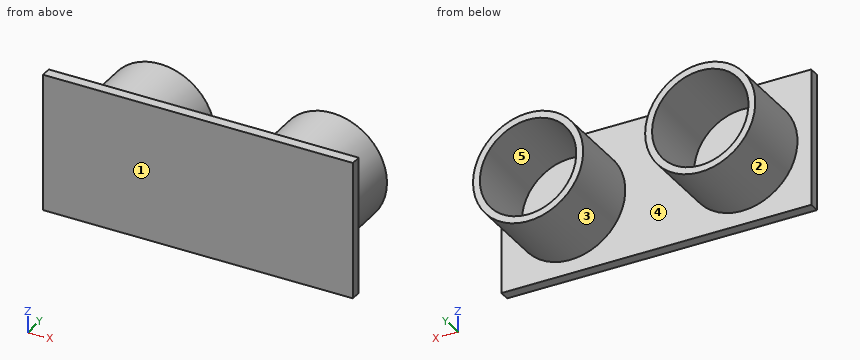
```python
from build123d import *

# Parameters (mm, degrees)
SKETCH1_W           = 45
SKETCH1_H           = 20
BOSS_EXTRUDE1_DEPTH = 1.5
SKETCH3_R           = 8
SKETCH3_R_2         = 7
BOSS_EXTRUDE2_DEPTH = 11


with BuildPart() as part:
    # Sketch1 → Boss-Extrude1 (new body)
    with BuildSketch(Plane(origin=(0, 0, 0), x_dir=(1, 0, 0), z_dir=(0, 1, 0))):
        Rectangle(SKETCH1_W, SKETCH1_H)
    extrude(amount=BOSS_EXTRUDE1_DEPTH)

    # Sketch3 → Boss-Extrude2 (add)
    with BuildSketch(Plane(origin=(0, 1.5, 0), x_dir=(1, 0, 0), z_dir=(0, 1, 0))):
        with Locations((-12.5, 0)):
            Circle(SKETCH3_R)
        with Locations((-12.5, 0)):
            Circle(SKETCH3_R_2, mode=Mode.SUBTRACT)
        with Locations((12.5, 0)):
            Circle(SKETCH3_R)
        with Locations((12.5, 0)):
            Circle(SKETCH3_R_2, mode=Mode.SUBTRACT)
    extrude(amount=BOSS_EXTRUDE2_DEPTH)


solid = part.part
```
Part model, mm, in its own coordinate system. Face numbers are marked on the shaded views. A direction names the side the tool comes from. Round coordinates to 2 decimals unless told otherwise and drop trailing zeros. Loops run counter-clockwise (first coordinate to the right, second up) from the corner with the lowest first, then second, coordinate; pieces in that order, holes last. Notation, with made-up numbers: (45.25, 24.25) -> (95.25, 24.25) arc R11 ccw to (95.25, 30.25) -> close; hole circle Ø8 at (9.25, -40). An arc over 180 degrees is marked (long way). Use a Markdown table: item, result.
1) Tool access for the marked faces 1 and 2: list every direction of +Z, -Z, +X, -X, +Y, -Y with a clear straight run to the whole face (end or side of a thin tool).
The answers:
| item | result |
|---|---|
| face 1 | +Z, -Z, +X, -X, -Y |
| face 2 | +Y |
2) Cut at C-C, the plane z = 0. List the corners of the cut face in (x, y).
The answers:
| item | result |
|---|---|
| outline | (-22.5, 0) -> (22.5, 0) -> (22.5, 1.5) -> (20.5, 1.5) -> (20.5, 12.5) -> (19.5, 12.5) -> (19.5, 1.5) -> (5.5, 1.5) -> (5.5, 12.5) -> (4.5, 12.5) -> (4.5, 1.5) -> (-4.5, 1.5) -> (-4.5, 12.5) -> (-5.5, 12.5) -> (-5.5, 1.5) -> (-19.5, 1.5) -> (-19.5, 12.5) -> (-20.5, 12.5) -> (-20.5, 1.5) -> (-22.5, 1.5) -> close |
3) Probe line 1 (X direction, y = 9.5, z = 0); line 2 (X direction, y = 2.5, z = -5.25); line 3 (Z direction, x = 12.5, y = 5.75). List the from-to ranges inside material, lowest first. Write a range as [from, to].
The answers:
| item | result |
|---|---|
| line 1 | x = [-20.5, -19.5], [-5.5, -4.5], [4.5, 5.5], [19.5, 20.5] |
| line 2 | x = [-18.54, -17.13], [-7.87, -6.46], [6.46, 7.87], [17.13, 18.54] |
| line 3 | z = [-8, -7], [7, 8] |
4) Pull direction Z, two halves, no side cores. Call the marked faces 3, 4 and 5: pulls with the +Z half, pulls with the -Z half, needs draft (parallel to the pull), parting line crosses it, or undercut.
The answers:
| item | result |
|---|---|
| face 3 | parting line crosses it |
| face 4 | needs draft |
| face 5 | undercut |
5) Cut at D-D, the plane z = -6. List the corners of the cut face in (x, y), and give its area (3 significant figures).
The answers:
| item | result |
|---|---|
| outline | (-22.5, 0) -> (22.5, 0) -> (22.5, 1.5) -> (17.79, 1.5) -> (17.79, 12.5) -> (16.11, 12.5) -> (16.11, 1.5) -> (8.89, 1.5) -> (8.89, 12.5) -> (7.21, 12.5) -> (7.21, 1.5) -> (-7.21, 1.5) -> (-7.21, 12.5) -> (-8.89, 12.5) -> (-8.89, 1.5) -> (-16.11, 1.5) -> (-16.11, 12.5) -> (-17.79, 12.5) -> (-17.79, 1.5) -> (-22.5, 1.5) -> close |
| area | 142 mm2 |
6) Drop flat-ended pins along their axis: pin 1 Ø7 at (x, z) = (13, -1.5) entering from +Y; pin 2 Ø3 at (x, y) = (-6.5, 6) entering from -Z. Give the stop position or say it passes through.
The answers:
| item | result |
|---|---|
| pin 1 | stops at y = 1.5 |
| pin 2 | stops at z = -6.61 |
7) Cut at B-B, the plane y = 11.5. List the corners of the cut face in (x, z).
The answers:
| item | result |
|---|---|
| outline | circle Ø16 at (-12.5, 0); circle Ø16 at (12.5, 0); hole circle Ø14 at (-12.5, 0); hole circle Ø14 at (12.5, 0) |
8) Cut at A-A, the plane x = -12.5. List the corners of the cut face in (y, z).
The answers:
| item | result |
|---|---|
| outline | (0, -10) -> (1.5, -10) -> (1.5, -8) -> (12.5, -8) -> (12.5, -7) -> (1.5, -7) -> (1.5, 7) -> (12.5, 7) -> (12.5, 8) -> (1.5, 8) -> (1.5, 10) -> (0, 10) -> close |
